Geometry check sheet. Reference: the model listing, model coordinates, mm. Face numbers are marked on the shaded views. A direction names the side the tool comes from. Give positions to 0.01 mm unless a question says otherwise; leave off trailing zeros. Order: outer loops, then holes, each group sorted by start corner. A loop starts at its lowest first (then second) coordinate and runs counter-clockwise, first axis right, second up.
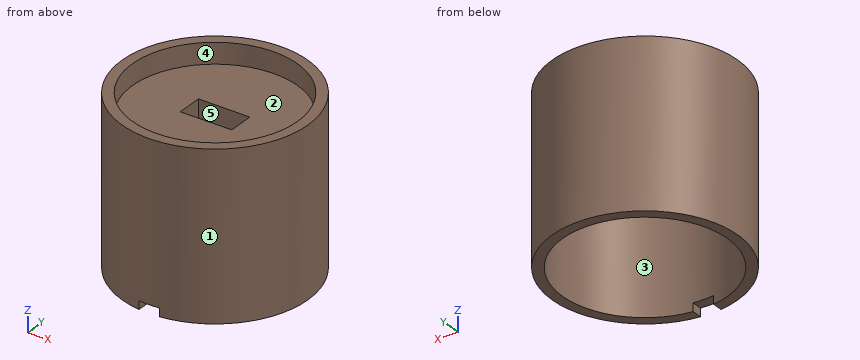
from build123d import *

# Parameters (mm, degrees)
F0_R     = 57.15
F1_DEPTH = 88.9
F2_R     = 50.8
F3_DEPTH = 76.2
F4_W     = 31.75
F4_H     = 15.875
F5_DEPTH = 12.7
F6_R     = 57.15
F6_R_2   = 50.8
F7_DEPTH = 12.7
F9_DEPTH = 5.08


with BuildPart() as f1:
    # F0 (on Top) → F1 (new body)
    with BuildSketch(Plane.XY):
        with Locations((-87.3053744435, 47.6011708379)):
            Circle(F0_R)
    extrude(amount=F1_DEPTH)

    # F2 (on face) → F3 (cut)
    with BuildSketch(Plane(origin=(0, 0, 0), x_dir=(1, 0, 0), z_dir=(0, 0, -1))):
        with Locations((-87.3053744435, -47.6011708379)):
            Circle(F2_R)
    extrude(amount=-F3_DEPTH, mode=Mode.SUBTRACT)

    # F4 (on face) → F5 (cut)
    with BuildSketch(Plane.XY.offset(88.9)):
        with Locations((-87.2800468532, 47.6297885038)):
            Rectangle(F4_W, F4_H)
    extrude(amount=-F5_DEPTH, mode=Mode.SUBTRACT)

    # F6 (on face) → F7 (join)
    with BuildSketch(Plane.XY.offset(88.9)):
        with Locations((-87.3053744435, 47.6011708379)):
            Circle(F6_R)
        with Locations((-87.3053744435, 47.6011708379)):
            Circle(F6_R_2, mode=Mode.SUBTRACT)
    extrude(amount=F7_DEPTH)

    # F8 (on face) → F9 (cut)
    with BuildSketch(Plane(origin=(0, 0, 0), x_dir=(1, 0, 0), z_dir=(0, 0, -1))):
        with BuildLine():
            ThreePointArc((-81.3538346767, 9.2380908956), (-87.7063174424, 9.5474227118), (-94.0538346767, 9.1489902586))
            Line((-94.0538346767, 9.1489902586), (-94.0538346767, 2.7485886897))
            ThreePointArc((-94.0538346767, 2.7485886897), (-87.7069848083, 3.1972416286), (-81.3538346767, 2.8489944186))
            Line((-81.3538346767, 2.8489944186), (-81.3538346767, 9.2380908956))
        make_face()
        with BuildLine():
            ThreePointArc((-81.3538346767, 2.8489944186), (-87.7069848083, 3.1972416286), (-94.0538346767, 2.7485886897))
            Line((-94.0538346767, 2.7485886897), (-94.0538346767, 0))
            Line((-94.0538346767, 0), (-81.3538346767, 0))
            Line((-81.3538346767, 0), (-81.3538346767, 2.8489944186))
        make_face()
    extrude(amount=-F9_DEPTH, mode=Mode.SUBTRACT)


solid = f1.part
Item 1: Sectioned sample at A-A (x = -97.5). Enter the section's corners in (y, z), and give its area (3 significant figures).
Reported:
outline: (-8.63, 0) - (-2.17, 0) - (-2.17, 76.2) - (39.69, 76.2) - (39.69, 88.9) - (-2.17, 88.9) - (-2.17, 101.6) - (-8.63, 101.6) - close; (55.57, 76.2) - (97.37, 76.2) - (97.37, 0) - (103.83, 0) - (103.83, 101.6) - (97.37, 101.6) - (97.37, 88.9) - (55.57, 88.9) - close
area: 2,380 mm2
Item 2: Sectioned sample at C-C (z = 84). Enter the section's corners in (x, y), and give its area (3 significant figures).
Reported:
outline: circle Ø114.3 at (-87.31, 47.6); hole (-103.16, 39.69) - (-71.41, 39.69) - (-71.41, 55.57) - (-103.16, 55.57) - close
area: 9,760 mm2
Item 3: Draft check along X on the marked faces 1 and 2. Enter one of: released by +X, released by -X, zero draft, split by the parting line, or undercut.
Reported:
face 1: split by the parting line
face 2: undercut
Item 4: Sectioned sample at D-D (x = -118.5). Enter the section's corners in (y, z), and give its area (3 significant figures).
Reported:
outline: (-0.28, 0) - (7.51, 0) - (7.51, 76.2) - (87.7, 76.2) - (87.7, 0) - (95.49, 0) - (95.49, 101.6) - (87.7, 101.6) - (87.7, 88.9) - (7.51, 88.9) - (7.51, 101.6) - (-0.28, 101.6) - close
area: 2,600 mm2
Item 5: Sectioned sample at B-B (y = 17.5). Enter the section's corners in (x, z), and give its area (3 significant figures).
Reported:
outline: (-135.89, 0) - (-128.23, 0) - (-128.23, 76.2) - (-46.38, 76.2) - (-46.38, 0) - (-38.73, 0) - (-38.73, 101.6) - (-46.38, 101.6) - (-46.38, 88.9) - (-128.23, 88.9) - (-128.23, 101.6) - (-135.89, 101.6) - close
area: 2,600 mm2
Item 6: Scan lines: L1, parallel to X at y = 76.5, z = 93.5; L2, parallel to Z at x = -86, y = 7; L3, parallel to Y at x = -107, z = 17.5. Record each from-to range of solid material in increasing order.
Reported:
L1: x = -136.61 to -129.08, -45.53 to -38
L2: z = 76.2 to 88.9
L3: y = -6.05 to 0.77, 94.43 to 101.25
Item 7: Set-up check for the marked faces 3, 4 and 5: record each of +Z, -Z, +X, -X, +Y, -Y from which the full face is reachable in a straight line by a thin tool's end or side.
Reported:
face 3: -Z
face 4: +Z
face 5: +Z, -Z
Item 8: Gauge pin test, flat ends, axial feed: pin 1 (1 mm diameter, centred on x = -106, z = 15, fed in from +Y); pin 2 (14 mm diameter, centred on y = 44.5, z = 83, fed in from +X); pin 3 (4 mm diameter, centred on x = -110, y = 52.5, fed in from -Z); pin 4 (1.5 mm diameter, centred on y = 74.5, z = 70, fed in from -X). Record the tip position at first contact, or that the pin passes through.
Reported:
pin 1: stops at y = 101.78
pin 2: stops at x = -30.16
pin 3: stops at z = 76.2
pin 4: stops at x = -138.12
